Check sheet for the drawn part. Datum: minimum x, y, z corner. Units: mm. Give positions to 0.01 mm unless a question says otherwise; leave off trailing zeros. Loops run counter-clockwise (first coordinate to the right, second up) from the corner with the lowest first, then second, coordinate; pieces in that order, holes last. Notation, with made-up numbers: (23.25, 53.25) - (46.25, 53.25) arc R35 ccw to (46.25, 90.25) - close; hole circle Ø6 at (21.5, -37). An arc over 180 degrees is marked (long way). One line per item, written item: value. Start each with the question number.
1. Scan lines: L1, parallel to Y at x = 28.5, z = 0.8; L2, parallel to Y at x = 4, z = 0.9. Record each from-to range of solid material in increasing order. Write a range as [from, to].
2. Sectioned sample at B-B (z = 0.8). Record the cut outline in (x, y), plus the area to 3 significant figures.
3. Mould release check, pull along Z, two halves, no side actions. Record for the marked faces 1 and 2: pulls with the +Z half, pulls with the -Z half, needs draft (parallel to the pull), parting line crosses it, or undercut.
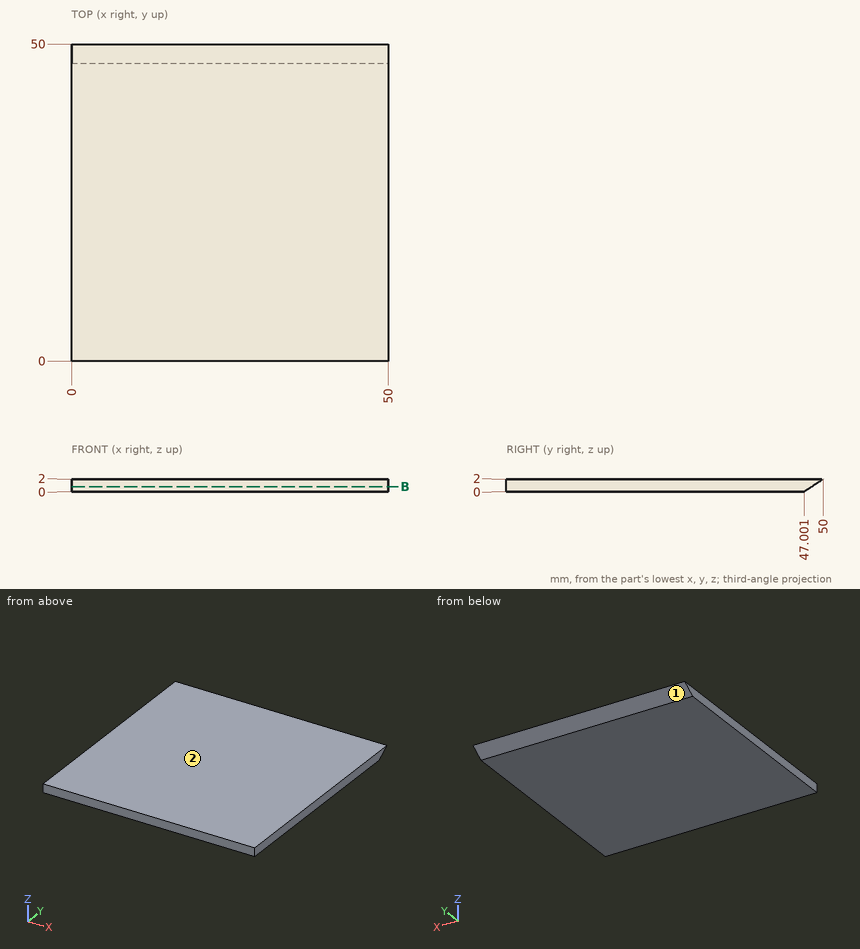
Results are:
1. L1: y = [0, 48.2]
1. L2: y = [0, 48.35]
2. outline: (0, 0) - (50, 0) - (50, 48.2) - (0, 48.2) - close
2. area: 2,410 mm^2
3. face 1: pulls with the -Z half
3. face 2: pulls with the +Z half
